Design review of the part shown in the three views and the two pictorial views. Dimensions are in mm from the part's minimum x, y and z. Coordinates: 2 decimals unless noted, no trailing zeros. Loops run counter-clockwise (first coordinate to the right, second up) from the corner with the lowest first, then second, coordinate; pieces in that order, holes last.
Q1. Add section B-B on z = 0.6. Give the number of separate pieces and of enclosed holes in the cut face, and give its area (3 significant figures).
Q2. Add section A-A on x = 25.4. Give the boundary of the cut face in (y, z) (1 decimal).
Q3. Add section C-C on y = 38.1. Give the boundary of the cut face in (x, z) (1 decimal).
Q4. Wall thickness on probe 1 along X at (y, z) = (88.9, 1.4); probe 2 along X at (y, z) = (40, 1.95) (1 decimal); probe 3 along Y at (x, z) = (139.7, 0.85): over which ranges is each line inside the solid? List them lowest first.
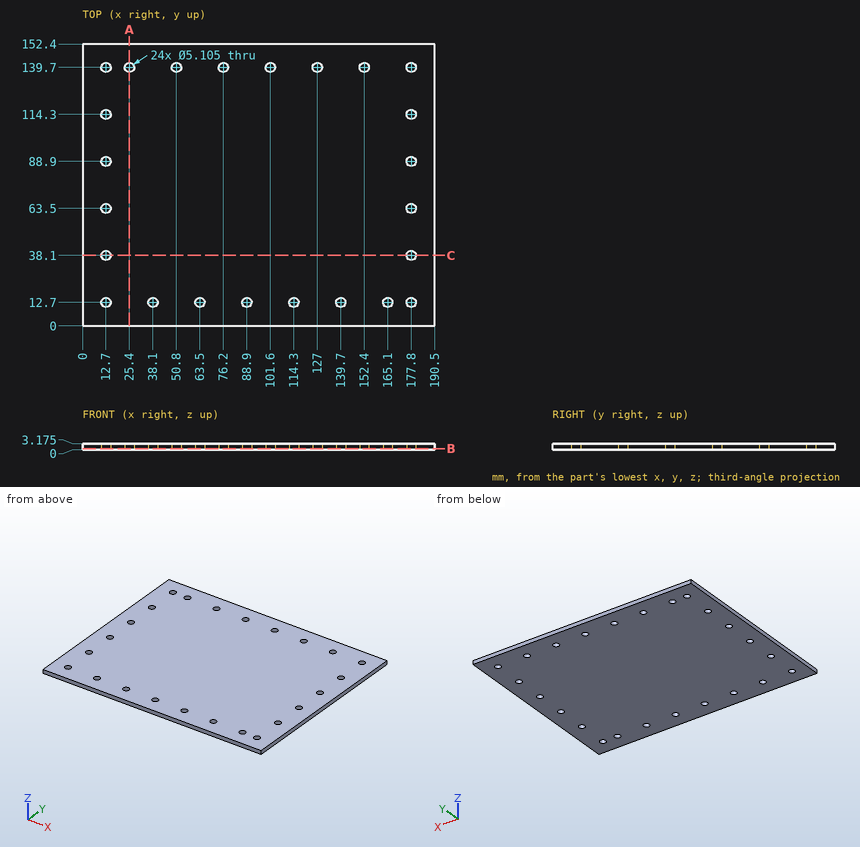
Entries:
1. separate pieces: 1
1. enclosed holes: 24
1. area: 28,500 mm2
2. outline: (0, 0) - (137.1, 0) - (137.1, 3.2) - (0, 3.2) - close; (142.3, 0) - (152.4, 0) - (152.4, 3.2) - (142.3, 3.2) - close
3. outline: (0, 0) - (10.1, 0) - (10.1, 3.2) - (0, 3.2) - close; (15.3, 0) - (175.2, 0) - (175.2, 3.2) - (15.3, 3.2) - close; (180.4, 0) - (190.5, 0) - (190.5, 3.2) - (180.4, 3.2) - close
4. probe 1: x = 0 to 10.15, 15.25 to 175.25, 180.35 to 190.5
4. probe 2: x = 0 to 11, 14.4 to 176.1, 179.5 to 190.5
4. probe 3: y = 0 to 10.15, 15.25 to 152.4
